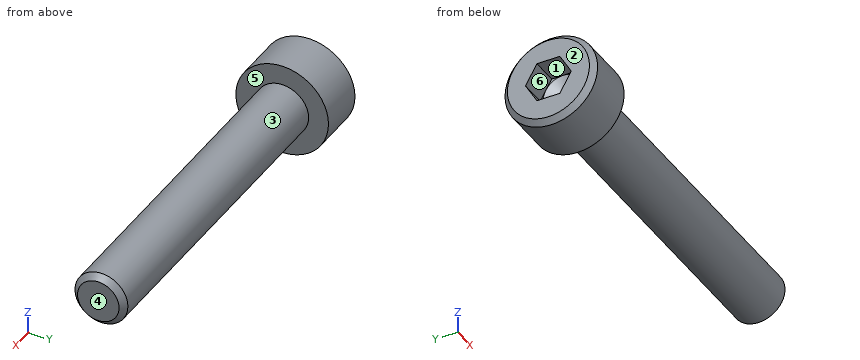
Autodesk Inventor part; units mm, degrees
ref_plane "bolt_to_nut_XY" through (25, 0, 0) normal (1, 0, 0) x (0, 0, -1)
ref_plane "bolt_to_nut_YZ" through (25, 0, 0) normal (0, 0, -1) x (0, 1, 0)
ref_plane "bolt_to_nut_ZX" through (25, 0, 0) normal (0, 1, 0) x (1, 0, 0)
sketch "Sketch_1" plane through (0, 0, 0) normal (0, 0, 1) x (1, 0, 0)
  line L0 (25, 0) -> (-4, 0)
  line L1 (-4, 0) -> (-4, 3.1)
  line L2 (-4, 3.1) -> (-3.6, 3.5)
  line L3 (-3.6, 3.5) -> (0, 3.5)
  line L4 (0, 3.5) -> (0, 2)
  line L5 (0, 2) -> (24.5705, 2)
  line L6 (24.5705, 2) -> (25, 1.5705)
  line L7 (25, 1.5705) -> (25, 0)
  line L8 (25, 0) -> (-4, 0)
revolve "Revolution1" add sketch "Sketch_1" angle 360 about axis through (25, 0, 0) along (1, 0, 0)
thread "Thread1"
sketch "Sketch_4_ALT_Drilling_1" plane through (0, 0, 0) normal (0, 0, 1) x (1, 0, 0)
  line L0 (-1.5981, 0) -> (-4, 0)
  line L1 (-4, 0) -> (-4, 1.5)
  line L2 (-4, 1.5) -> (-2, 1.5)
  line L3 (-2, 1.5) -> (-1.5981, 0)
  line L4 (-1.5981, 0) -> (-4, 0)
revolve "Revolution2" cut sketch "Sketch_4_ALT_Drilling_1" angle 360 about axis through (-1.5981, 0, 0) along (1, 0, 0)
sketch "Sketch_3" plane through (-4, 0, 0) normal (1, 0, 0) x (0, 0, -1)
  line L0 (-1.5, -0.866) -> (0, -1.7321)
  line L1 (0, -1.7321) -> (1.5, -0.866)
  line L2 (1.5, -0.866) -> (1.5, 0.866)
  line L3 (1.5, 0.866) -> (0, 1.7321)
  line L4 (0, 1.7321) -> (-1.5, 0.866)
  line L5 (-1.5, 0.866) -> (-1.5, -0.866)
extrude "Extrusion1" cut sketch "Sketch_3" along normal blind 2
ref_plane "bolt_to_nut_XY" through (25, 0, 0) normal (1, 0, 0) x (0, 0, -1)
ref_plane "bolt_to_nut_YZ" through (25, 0, 0) normal (0, 0, -1) x (0, 1, 0)
ref_plane "bolt_to_nut_ZX" through (25, 0, 0) normal (0, 1, 0) x (1, 0, 0)
ref_plane "screw1_XY" through (0, 0, 0) normal (1, 0, 0) x (0, 0, -1)
ref_plane "screw1_YZ" through (0, 0, 0) normal (0, 0, -1) x (0, 1, 0)
ref_plane "screw1_ZX" through (0, 0, 0) normal (0, 1, 0) x (1, 0, 0)
properties part number "CB4-25" material "鋼、炭素鋼"
Part model, mm, in its own coordinate system. Face numbers are marked on the shaded views. A direction names the side the tool comes from. Give positions to 0.01 mm unless a question says otherwise; leave off trailing zeros. Order: outer loops, then holes, each group sorted by start corner. A loop starts at its lowest first (then second) coordinate and runs counter-clockwise, first axis right, second up. Notation, with made-up numbers: (64, 86) - (111, 86) arc R20 ccw to (111, 119) - close; hole circle Ø4 at (24, -31). An arc over 180 degrees is marked (long way). Use one line per item in the form item = value.
Item 1: Pin check, flat tips, straight feed: pin 1 Ø1 at (x, y) = (4, -1) entering from -Z; pin 2 Ø0.9 at (y, z) = (-0.5, 0) entering from -X; pin 3 Ø0.5 at (x, y) = (-2.5, -0.5) entering from -Z. Stop position of each tip, or through.
Solution:
pin_1 = -1.94
pin_2 = -1.85
pin_3 = -3.49
Item 2: Slice it at A-A on x = 3.5. Give the cut face in (y, z).
Solution:
outline = circle Ø4 at (0, 0)
Item 3: Probe probe 1 along X at (y, z) = (0, -0.5); probe 2 along Z at (x, y) = (22.75, 0); probe 3 along Y at (x, z) = (16, 1). List the from-to ranges inside material, lowest first. Write a range as from..to.
Solution:
probe_1 = -1.73..25
probe_2 = -2..2
probe_3 = -1.73..1.73
Item 4: Which spindle directions (+Z, -Z, +X, -X, +Y, -Y) get a long thin tool onto all of the face, cutting with end or side? Do the marked faces 4, 5 and 6. Say none if no direction does.
Solution:
face_4 = +Z, -Z, +X, +Y, -Y
face_5 = +X
face_6 = -X
Item 5: Two-plate mould, pull along Z, no slides. Class the marked faces 1, 2 and 3: released by +Z, released by -Z, zero draft, split by the parting line, or undercut.
Solution:
face_1 = undercut
face_2 = zero draft
face_3 = split by the parting line
